Source: CAD feature listing. Evaluate the final solid. Frame: model axes, mm. Give positions to 0.01 mm unless a question says otherwise; leave off trailing zeros. Write each loop counter-clockwise with the first axis right and the second up, starting at its lowest first coordinate (ties: lowest second). Pieces come first, ordered by that corner, then holes.
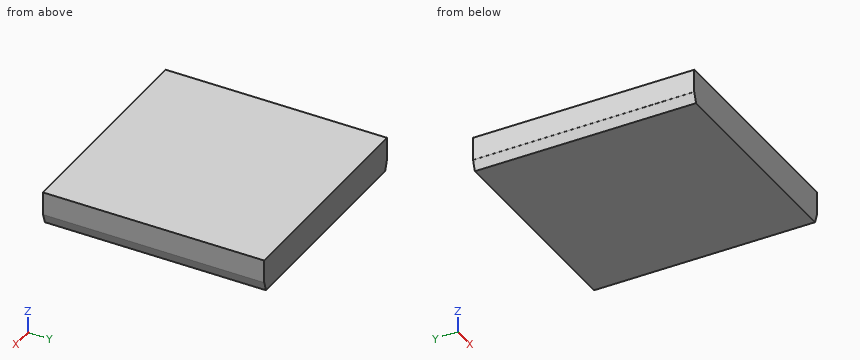
Autodesk Inventor part; units mm, degrees
ref_plane "YZ Plane" through (0, 0, 0) normal (1, 0, 0) x (0, 1, 0)
ref_plane "XZ Plane" through (0, 0, 0) normal (0, 1, 0) x (-1, 0, 0)
ref_plane "XY Plane" through (0, 0, 0) normal (0, 0, 1) x (1, 0, 0)
sketch "草图1" plane through (0, 0, 0) normal (0, 0, 1) x (1, 0, 0)
  line L0 (485, -500) -> (-485, -500)
  line L1 (-485, -500) -> (-485, 500)
  line L2 (-485, 500) -> (485, 500)
  line L3 (485, 500) -> (485, -500)
  line L4 (485, -500) -> (-485, 500) construction
  line L5 (-485, -500) -> (485, 500) construction
  point P0 (0, 0)
  dimension "d0" = 1000
  dimension "d1" = 970
extrude "拉伸1" add sketch "草图1" along normal blind 45
sketch "草图2" plane through (0, 0, 45) normal (0, 0, 1) x (1, 0, 0)
  line L0 (500, -500) -> (-500, -500)
  line L1 (-500, -500) -> (-500, 500)
  line L2 (-500, 500) -> (500, 500)
  line L3 (500, 500) -> (500, -500)
  line L4 (500, -500) -> (-500, 500) construction
  line L5 (-500, -500) -> (500, 500) construction
  line L6 (485, 500) -> (-485, 500)
  line L7 (-485, 500) -> (-485, -500)
  point P0 (0, 0)
  point P1 (-485, 500)
  dimension "d5" = 1000
extrude "拉伸2" add sketch "草图2" along normal blind 105
chamfer "倒角1" distance 14.5 distance2 45 1 edges at (-485, 0, 45) measured on face at (-490, 166.6667, 45)
chamfer "倒角2" distance 14.75 distance2 44.75 1 edges at (485, 0, 45) measured on face at (495, 166.6667, 45)
1. Line query: probe 1 along X at (y, z) = (158, 36); probe 2 along X at (y, z) = (172.5, 38.5). Output: solid intervals per line, ascending.
2. Section query A-A (z = 13.5). Return loops of the section in (x, y), plus the area to 3 significant figures.
3. Pin query (flat end, axial travel): P1, Ø5, axis at y = 173.5, z = 41, coming from the +X side. Return the tip coordinate at first contact, or that it passes through.
The answers:
1. probe 1: x = -496.6 to 496.78
1. probe 2: x = -497.41 to 497.61
2. outline: (-489.35, -500) - (489.37, -500) - (489.37, 500) - (-489.35, 500) - close
2. area: 979,000 mm2
3. P1: stops at x = 499.26
